Source: three-view drawing plus pictorial views. Frame: mm from the lowest corner of the part. A direction names the side the tool comes from. Give positions to 0.01 mm unless a question says otherwise; leave off trailing zeros. Order: outer loops, then holes, each group sorted by start corner. A loop starts at its lowest first (then second) coordinate and runs counter-clockwise, first axis right, second up. Notation, with made-up numbers: M 32.25,26 L 82.25,26 A21 cw 82.25,49 Z; hole C -22.5,78 d10. An arc over 180 degrees is marked long. Use CSV: the item, a comma, the result in double quotes. Start each with the question number.
1. Reachability of the marked faces 5, 6 and 7 from +Z, -Z, +X, -X, +Y, -Y: full face, straight path, thin tool, end or side. Return the list, or none.
2. Pin query (flat end, axial travel): P1, Ø2.5, axis at x = 7, y = 5, coming from the -Z side; P2, Ø5, axis at x = 5.5, z = 15, coming from the -Y side; P3, Ø2, axis at y = 5, z = 13, coming from the +X side; P4, Ø0.5, axis at x = 18.5, y = 4.5, coming from the -Z side. Return the tip coordinate at first contact, or that it passes through.
3. Section query A-A, the plane z = 13.5. Return the cut outline in (x, y), plus the area to 3 significant figures.
4. Mould query, pull axis Z, two halves, no side actions, for the marked faces 1, 2, 3 and 4. Classes: released by +Z, released by -Z, zero draft, split by the parting line, or undercut.
5. Section query B-B, the plane x = 4. Return the cut outline in (y, z).
6. Line query: line 1 along X through (y, z) = (9.7, 4); line 2 along Y through (x, z) = (16.75, 16.5); line 3 along Y through (x, z) = (8.25, 9.5). Output: solid intervals per line, ascending. Write a range as [from, to].
7. Section query D-D, the plane z = 4. Return the cut outline in (x, y), plus the area to 3 significant figures.
8. Section query C-C, the plane y = 4. Return the cut outline in (x, z).
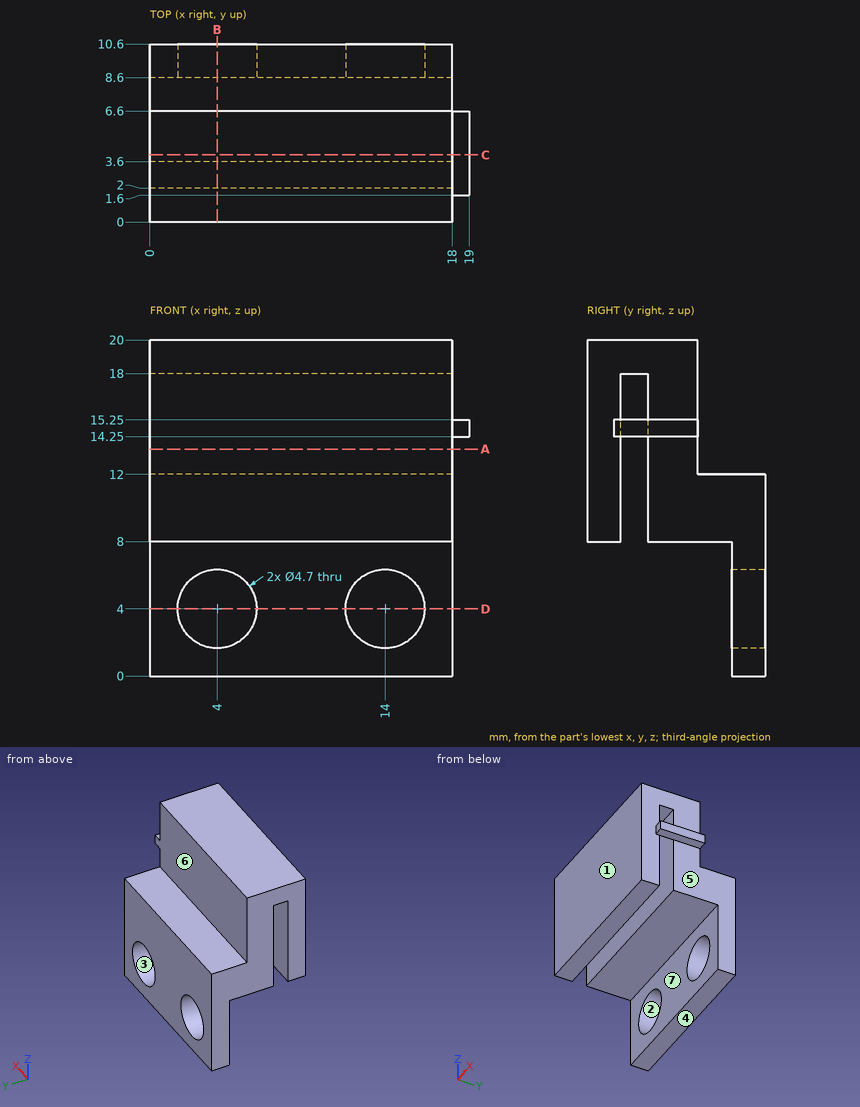
Result set:
1,face 5,"-Z, +X, +Y, -Y"
1,face 6,"+Z, +X, -X, +Y"
1,face 7,"-Z, +X, -X, -Y"
2,P1,"z = 8"
2,P2,"y = 0"
2,P3,"x = 18"
2,P4,"z = 14.25"
3,outline,"M 0,0 L 18,0 L 18,2 L 0,2 Z; M 0,3.6 L 18,3.6 L 18,6.6 L 0,6.6 Z"
3,area,"90.0 mm2"
4,face 1,"zero draft"
4,face 2,"undercut"
4,face 3,"undercut"
4,face 4,"released by -Z"
5,outline,"M 0,8 L 2,8 L 2,18 L 3.6,18 L 3.6,8 L 8.6,8 L 8.6,6.35 L 10.6,6.35 L 10.6,12 L 6.6,12 L 6.6,20 L 0,20 Z; M 8.6,0 L 10.6,0 L 10.6,1.65 L 8.6,1.65 Z"
6,line 1,"[0, 1.65], [6.35, 11.65], [16.35, 18]"
6,line 2,"[0, 2], [3.6, 6.6]"
6,line 3,"[0, 2], [3.6, 10.6]"
7,outline,"M 0,8.6 L 1.65,8.6 L 1.65,10.6 L 0,10.6 Z; M 6.35,8.6 L 11.65,8.6 L 11.65,10.6 L 6.35,10.6 Z; M 16.35,8.6 L 18,8.6 L 18,10.6 L 16.35,10.6 Z"
7,area,"17.2 mm2"
8,outline,"M 0,8 L 18,8 L 18,14.25 L 19,14.25 L 19,15.25 L 18,15.25 L 18,20 L 0,20 Z"
